```python
from build123d import *

# Parameters (mm, degrees)
SKETCH1_W            = 155
SKETCH1_H            = 77
BOSS_EXTRUDE1_DEPTH  = 1.6
SKETCH2_R            = 3.47579735
BOSS_EXTRUDE3_DEPTH  = 5
M2_CLEARANCE_HOLE1_D = 2.2


with BuildPart() as part:
    # Sketch1 → Boss-Extrude1 (new body)
    with BuildSketch(Plane(origin=(0, 0, 0), x_dir=(1, 0, 0), z_dir=(0, 1, 0))):
        with Locations((77.5, -38.5)):
            Rectangle(SKETCH1_W, SKETCH1_H)
    extrude(amount=BOSS_EXTRUDE1_DEPTH)

    # Sketch2 → Boss-Extrude3 (add)
    with BuildSketch(Plane(origin=(0, 1.6, 0), x_dir=(1, 0, 0), z_dir=(0, 1, 0))):
        with Locations(Location((63.398865642, -16.538313278, 0), (0, 0, 270))):
            Circle(SKETCH2_R)
        with Locations(Location((63.398865642, -44.168086722, 0), (0, 0, 270))):
            Circle(SKETCH2_R)
        with Locations(Location((149.449734358, -16.538313278, 0), (0, 0, 270))):
            Circle(SKETCH2_R)
        with Locations(Location((149.449734358, -44.168086722, 0), (0, 0, 270))):
            Circle(SKETCH2_R)
    extrude(amount=BOSS_EXTRUDE3_DEPTH)

    # M2 Clearance Hole1 (through all)
    with Locations(Plane(origin=(0, 1.6, 0), x_dir=(1, 0, 0), z_dir=(0, 1, 0))):
        with Locations((147.994644581, -5.281684189), (147.994644581, -72.114274551), (57.497596152, -72.114274551), (57.497596152, -5.281684189)):
            Hole(M2_CLEARANCE_HOLE1_D / 2)


solid = part.part
```
Here's how the part is built. I have some questions about the finished solid (model axes, mm). A direction names the side the tool comes from. Give positions to 0.01 mm unless a question says otherwise; leave off trailing zeros. Write each loop counter-clockwise with the first axis right and the second up, starting at its lowest first coordinate (ties: lowest second). Pieces come first, ordered by that corner, then holes.
(1) Imagine slicing it at B-B, the plane z = 58.5. Write out the boundary of the cut face in (x, y).
Output values:
outline: (0, 0) - (155, 0) - (155, 1.6) - (0, 1.6) - close
(2) On a 3-axis mill with a long thin cutter (end or side, diameter ignored), from which of +Z, -Z, +X, -X, +Y, -Y can I reach the whole of each face in a straight line? I mean faces 3 (the face through (66.33, 4.065, 46.037)), 4 (the face through (149, 6.6, 44)). Say none if no direction works.
Output values:
face 3: +Y
face 4: +Z, -Z, +X, -X, +Y
(3) Imagine slicing it at A-A, the plane x = 137. Write out the boundary of the cut face in (y, z), and give its area (3 significant figures).
Output values:
outline: (0, 0) - (1.6, 0) - (1.6, 77) - (0, 77) - close
area: 123 mm2
(4) Thinking about a two-plate mould opening in Z: for faces 1 (the face through (63, 6.6, 16)), 2 (the face through (66.33, 4.06, 18.41)), which applies, pulls with the +Z half, pulls with the -Z half, needs draft (parallel to the pull), parting line crosses it, or undercut?
Output values:
face 1: needs draft
face 2: undercut
(5) Will these pins go through, and if not, where does the flat tip stop? pin 1 (23 mm diameter, centred on x = 45.5, z = 41, fed in from +Y); pin 2 (1 mm diameter, centred on y = 2.5, z = 65.5, fed in from -X).
Output values:
pin 1: stops at y = 1.6
pin 2: passes through
(6) Imagine slicing it at D-D, the plane z = 46. Write out the boundary of the cut face in (x, y), and give its area (3 significant figures).
Output values:
outline: (0, 0) - (155, 0) - (155, 1.6) - (152.4, 1.6) - (152.4, 6.6) - (146.5, 6.6) - (146.5, 1.6) - (66.35, 1.6) - (66.35, 6.6) - (60.45, 6.6) - (60.45, 1.6) - (0, 1.6) - close
area: 307 mm2
(7) Imagine slicing it at C-C, the plane y = 5. Write out the boundary of the cut face in (x, z), and give its area (3 significant figures).
Output values:
outline: circle Ø6.95 at (63.4, 16.54); circle Ø6.95 at (63.4, 44.17); circle Ø6.95 at (149.45, 16.54); circle Ø6.95 at (149.45, 44.17)
area: 152 mm2
(8) If I drill on L1, parallel to X at y = 4, z = 44; L2, parallel to Y at x = 101.5, z = 59; L3, parallel to Z at x = 147, y = 6.25, over which ranges is the centre line in solid material (lowest first)?
Output values:
L1: x = 59.93 to 66.87, 145.98 to 152.92
L2: y = 0 to 1.6
L3: z = 14.07 to 19, 41.7 to 46.63
